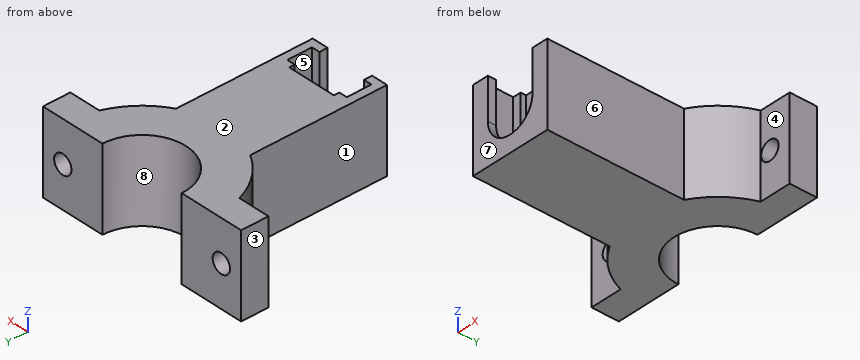
Autodesk Inventor part; units mm, degrees
ref_plane "YZ Plane" through (0, 0, 0) normal (1, 0, 0) x (0, 1, 0)
ref_plane "XZ Plane" through (0, 0, 0) normal (0, 1, 0) x (-1, 0, 0)
ref_plane "XY Plane" through (0, 0, 0) normal (0, 0, 1) x (1, 0, 0)
sketch "Sketch1" plane through (0, 0, 0) normal (0, 0, 1) x (1, 0, 0)
  line L0 (0, 0) -> (15, 0)
  line L1 (15, 0) -> (15, 30)
  line L2 (15, 30) -> (0, 30)
  line L3 (0, 30) -> (0, 0)
  line L4 (7.5, 30) -> (7.5, 38)
  arc A0 (-0.5, 38) -> (15.5, 38) centre (7.5, 38) ccw
  arc A1 (-7.5, 38) -> (22.5, 38) centre (7.5, 38) ccw
  line L5 (-0.5, 38) -> (-7.5, 38)
  line L6 (15.5, 38) -> (22.5, 38)
  line L7 (22.5, 38) -> (27.5, 38)
  line L8 (27.5, 38) -> (27.5, 33)
  line L9 (27.5, 33) -> (21.6421, 33)
  line L10 (-7.5, 38) -> (-12.5, 38)
  line L11 (-12.5, 38) -> (-12.5, 33)
  line L12 (-12.5, 33) -> (-6.6421, 33)
  dimension "d0" = 15
  dimension "d1" = 30
  dimension "d2" = 8
  dimension "d3" = 16
  dimension "d4" = 30
  dimension "d5" = 5
  dimension "d6" = 5
  dimension "d7" = 5
  dimension "d8" = 5
extrude "Extrusion1" add sketch "Sketch1" along normal blind 15
sketch "Sketch2" plane through (0, 0, 15) normal (0, 0, 1) x (1, 0, 0)
  line L0 (0, 0) -> (15, 0)
  line L1 (7.5, 0) -> (3, 0)
  line L2 (3, 0) -> (3, 1.5)
  line L3 (3, 1.5) -> (1.5, 1.5)
  line L4 (1.5, 1.5) -> (1.5, 6)
  line L5 (1.5, 6) -> (3, 6)
  line L6 (3, 6) -> (3, 7)
  line L7 (7.5, 0) -> (12, 0)
  line L8 (12, 0) -> (12, 1.5)
  line L9 (12, 1.5) -> (13.5, 1.5)
  line L10 (13.5, 1.5) -> (13.5, 6)
  line L11 (13.5, 6) -> (12, 6)
  line L12 (12, 6) -> (12, 7)
  line L13 (12, 7) -> (3, 7)
  dimension "d11" = 4.5
  dimension "d12" = 1.5
  dimension "d13" = 1.5
  dimension "d14" = 4.5
  dimension "d15" = 1.5
  dimension "d16" = 1
  dimension "d17" = 4.5
  dimension "d18" = 1.5
sketch "Sketch3" plane through (0, 0, 0) normal (0, -1, 0) x (1, 0, 0)
  line L0 (-0.5, 15) -> (15.5, 15)
  line L1 (7.5, 15) -> (7.5, 7.5)
  circle A0 centre (7.5, 7.5) radius 4.5
  point P0 (0, 0)
  dimension "d19" = 7.5
  dimension "d20" = 9
extrude "Extrusion2" cut sketch "Sketch3" against normal blind 1.5
sketch "Sketch4" plane through (7.5, 1.5, 7.5) normal (0, -1, 0) x (1, 0, 0)
  point P0 (-7.5, -7.5)
extrude "Extrusion3" cut sketch "Sketch2" against normal blind 7.5
sketch "Sketch5" plane through (0, 0, 7.5) normal (0, 0, 1) x (1, 0, 0)
  line L0 (13.5, 6) -> (13.5, 1.5)
  line L1 (3, 1.5) -> (1.5, 1.5)
  line L2 (13.5, 1.5) -> (1.5, 1.5)
  line L3 (1.5, 1.5) -> (1.5, 6)
  line L4 (1.5, 1.5) -> (1.5, 6)
  line L5 (1.5, 6) -> (3, 6)
  line L6 (1.5, 6) -> (3, 6)
  line L7 (3, 7) -> (12, 7)
  line L8 (3, 6) -> (3, 7)
  line L9 (3, 7) -> (12, 7)
  line L10 (12, 6) -> (13.5, 6)
  line L11 (12, 7) -> (12, 6)
  line L12 (12, 6) -> (13.5, 6)
  line L13 (13.5, 6) -> (13.5, 1.5)
  point P0 (0, 0)
extrude "Extrusion4" cut sketch "Sketch5" against normal blind 5
sketch "Sketch6" plane through (-12.5, 38, 0) normal (0, 1, 0) x (1, 0, 0)
  line L0 (0, 0) -> (0, -15)
  line L1 (0, -7.5) -> (4, -7.5)
  line L2 (40, 0) -> (40, -15)
  line L3 (40, -7.5) -> (36, -7.5)
  circle A0 centre (4, -7.5) radius 1.75
  circle A1 centre (36, -7.5) radius 1.75
  point P0 (12.5, 0)
  dimension "d27" = 4
  dimension "d28" = 4
  dimension "d29" = 3.5
  dimension "d30" = 3.5
extrude "Extrusion5" cut sketch "Sketch6" against normal through all
properties part number "prism_holder_1"
Check sheet for the modelled part. Datum: model origin and axes. Units: mm. Face numbers are marked on the shaded views. A direction names the side the tool comes from. Coordinates: 2 decimals unless noted, no trailing zeros. Write each loop counter-clockwise with the first axis right and the second up, starting at its lowest first coordinate (ties: lowest second). Pieces come first, ordered by that corner, then holes. Notation, with made-up numbers: M -26,21.5 L 13,21.5 A25 cw 13,60.5 Z; hole C 66,23.25 d8. An arc over 180 degrees is marked long. Answer as CSV lines item,"result".
Q1. Cross-section at C-C (x = 7.5). Record the boundary of the cut face in (y, z), then the cut area to 3 significant figures.
Check result:
outline,"M 0,0 L 30,0 L 30,15 L 7,15 L 7,2.5 L 1.5,2.5 L 1.5,3 L 0,3 Z"
area,"363 mm^2"
Q2. Material ranges on probe 1 along Z at (x, y) = (-8.5, 35.1); probe 2 along X at (y, z) = (36.25, 7.5); probe 3 along X at (y, z) = (7, 0.75), recorded low to high. Write a range as from..to.
Check result:
probe 1,"0..5.75, 9.25..15"
probe 2,"-12.5..-10.25, -6.75..-0.31, 15.31..21.75, 25.25..27.5"
probe 3,"0..15"
Q3. Set-up check for the marked faces 1, 2, 3, 4 and 5: record each of +Z, -Z, +X, -X, +Y, -Y from which the full face is reachable in a straight line by a thin tool's end or side.
Check result:
face 1,"+Z, -Z, -X, -Y"
face 2,"+Z, +X, -X, +Y, -Y"
face 3,"+Z, -Z, -X, +Y, -Y"
face 4,"+Z, -Z, +X, -Y"
face 5,"+Z"
Q4. Cross-section at D-D (z = 8.75). Count the separate pieces of the cut face and the enclosed holes in it, then the cut area to 3 significant figures.
Check result:
separate pieces,"3"
enclosed holes,"0"
area,"559 mm^2"
Q5. Go/stop test with flat-tipped pins: pin 1 (7.5 mm diameter, centred on y = 12.5, z = 6, fed in from +X); pin 2 (2.5 mm diameter, centred on x = 7.5, z = 6.5, fed in from -Y); pin 3 (4 mm diameter, centred on y = 8.5, z = 7, fed in from -X). Record where each tip stops, or that it passes through.
Check result:
pin 1,"x = 15"
pin 2,"y = 7"
pin 3,"x = 0"
Q6. Cross-section at B-B (y = 35). Record the boundary of the cut face in (x, z).
Check result:
outline,"M -12.5,0 L 0.08,0 L 0.08,15 L -12.5,15 Z; M 14.92,0 L 27.5,0 L 27.5,15 L 14.92,15 Z; hole C -8.5,7.5 d3.5; hole C 23.5,7.5 d3.5"
Q7. Cross-section at A-A (x = 23.5). Record the boundary of the cut face in (y, z), then the cut area to 3 significant figures.
Check result:
outline,"M 33,0 L 38,0 L 38,5.75 L 33,5.75 Z; M 33,9.25 L 38,9.25 L 38,15 L 33,15 Z"
area,"57.5 mm^2"
Q8. Mould release check, pull along X, two halves, no side actions. Record for the marked faces 6, 7 and 8: released by +X, released by -X, zero draft, split by the parting line, or undercut.
Check result:
face 6,"released by +X"
face 7,"zero draft"
face 8,"undercut"
